Verification items for the finished model (mm, model axes). Face numbers are marked on the shaded views. Coordinates: 2 decimals unless noted, no trailing zeros. Loops run counter-clockwise (first coordinate to the right, second up) from the corner with the lowest first, then second, coordinate; pieces in that order, holes last. Notation, with made-up numbers: (-14, 32) -> (25, 32) arc R31 cw to (25, 59) -> close; hole circle Ø11 at (80.5, 54.5). An arc over 180 degrees is marked (long way). Answer as a JSON object with one key per item and string values. Group by question number.
Q1. Cross-section at A-A on z = 2.75. Record the boundary of the cut face in (x, y).
Q2. Scan lines: L1, parallel to Y at x = 18, z = 1.15; L2, parallel to X at y = 22.5, z = 3.6; L3, parallel to Y at x = 43, z = 0.8. Record each from-to range of solid material in increasing order.
Q3. Gauge pin test, flat ends, axial feed: pin 1 Ø2.5 at (x, z) = (-25, 1.5) entering from +Y; pin 2 Ø1.5 at (x, z) = (20.5, 3.5) entering from -Y; pin 3 Ø1 at (y, z) = (20, 4.5) entering from +X. Record the tip position at first contact, or that the pin passes through.
Q4. Release check for a two-part mould opening along Z. For the marked faces 1 and 2 record: released by +Z, released by -Z, zero draft, split by the parting line, or undercut.
Q5. Cross-section at B-B on y = 15. Record the boundary of the cut face in (x, z).
Q6. Cross-section at D-D on x = -20. Record the boundary of the cut face in (y, z).
Q7. Cross-section at C-C on x = -46.5. Record the boundary of the cut face in (y, z).
```python
from build123d import *

# Parameters (mm, degrees)
F1_DEPTH = 5.08


with BuildPart() as f1:
    # F0 (on Top) → F1 (new body)
    with BuildSketch(Plane.XY):
        Polygon((-30.73996, 53.627926), (-62.727489, 79.665363), (-37.928027, 48.796157), (-31.880961, 41.269053), (-17.285284, 23.101039), (-40.998805, 23.101039), (-2.661946, -15.828654), (-29.339654, -15.828654), (29.78309, -64.496771), (38.018424, -71.275857), (67.885771, -95.861785), (45.034323, -67.141476), (39.001086, -59.558743), (23.094157, -39.566491), (47.522068, -39.566491), (8.569453, 0), (35.143055, 0), (-22.663309, 47.053636), align=None)
        with BuildLine():
            Line((-31.880961, 41.269053), (-37.928027, 48.796157))
            ThreePointArc((-37.928027, 48.796157), (-54.894131, -45.989389), (38.018424, -71.275857))
            Line((38.018424, -71.275857), (29.78309, -64.496771))
            ThreePointArc((29.78309, -64.496771), (-47.893768, -38.925538), (-31.880961, 41.269053))
        make_face()
        with BuildLine():
            ThreePointArc((45.034323, -67.141476), (65.788888, 30.03676), (-30.73996, 53.627926))
            Line((-30.73996, 53.627926), (-22.663309, 47.053636))
            ThreePointArc((-22.663309, 47.053636), (58.757468, 23.007783), (39.001086, -59.558743))
            Line((39.001086, -59.558743), (45.034323, -67.141476))
        make_face()
    extrude(amount=F1_DEPTH)


solid = f1.part
```
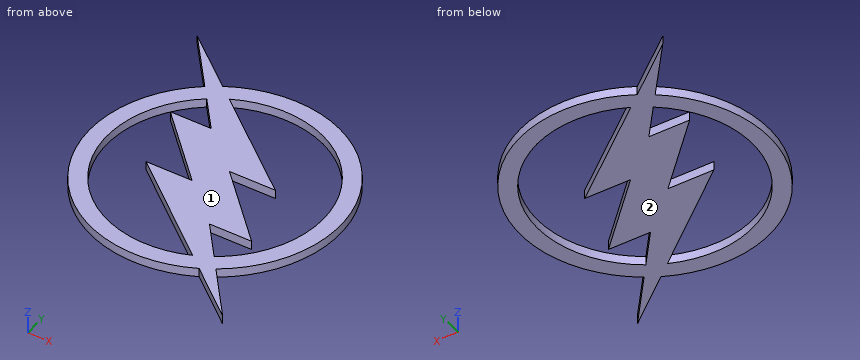
Computed values:
{
 "1": {"outline": "(-62.73, 79.67) -> (-37.93, 48.8) arc R71.32 ccw to (38.02, -71.28) -> (67.89, -95.86) -> (45.03, -67.14) arc R71.32 ccw to (-30.74, 53.63) -> close; hole (-41, 23.1) -> (-17.29, 23.1) -> (-31.88, 41.27) arc R61.66 ccw to (29.78, -64.5) -> (-29.34, -15.83) -> (-2.66, -15.83) -> close; hole (-22.66, 47.05) -> (35.14, 0) -> (8.57, 0) -> (47.52, -39.57) -> (23.09, -39.57) -> (39, -59.56) arc R61.66 ccw to start"},
 "2": {"L1": "y = -78.06 to -68.23, -54.8 to -9.58, 0 to 13.95, 52.49 to 62.32", "L2": "x = -59.15 to -48.29, -40.41 to 7.5, 59.05 to 69.91", "L3": "y = -75.38 to -56.73, -39.57 to -34.97, 40.99 to 52.72"},
 "3": {"pin 1": "stops at y = 57.23", "pin 2": "stops at y = -77.72", "pin 3": "stops at x = 71.24"},
 "4": {"face 1": "released by +Z", "face 2": "released by -Z"},
 "5": {"outline": "(-62.17, 0) -> (-51.89, 0) -> (-51.89, 5.08) -> (-62.17, 5.08) -> close; (-33.02, 0) -> (16.72, 0) -> (16.72, 5.08) -> (-33.02, 5.08) -> close; (62.65, 0) -> (72.93, 0) -> (72.93, 5.08) -> (62.65, 5.08) -> close"},
 "6": {"outline": "(-74.52, 0) -> (-64.07, 0) -> (-64.07, 5.08) -> (-74.52, 5.08) -> close; (-23.52, 0) -> (-15.83, 0) -> (-15.83, 5.08) -> (-23.52, 5.08) -> close; (1.78, 0) -> (23.1, 0) -> (23.1, 5.08) -> (1.78, 5.08) -> close; (26.48, 0) -> (44.89, 0) -> (44.89, 5.08) -> (26.48, 5.08) -> close; (48.33, 0) -> (58.78, 0) -> (58.78, 5.08) -> (48.33, 5.08) -> close"},
 "7": {"outline": "(-56.8, 0) -> (-41.2, 0) -> (-41.2, 5.08) -> (-56.8, 5.08) -> close; (25.47, 0) -> (41.07, 0) -> (41.07, 5.08) -> (25.47, 5.08) -> close; (59.47, 0) -> (66.46, 0) -> (66.46, 5.08) -> (59.47, 5.08) -> close"}
}
